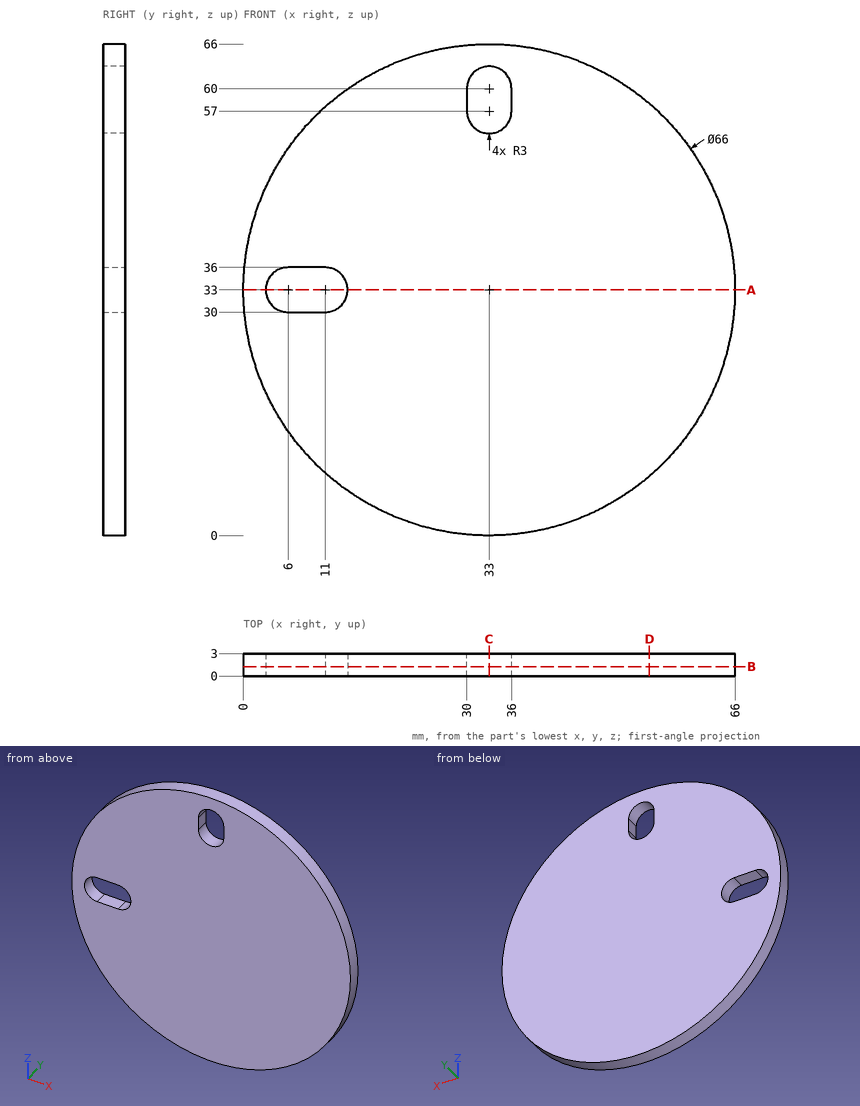
Geometry check sheet. Reference: drawing and pictorial views, mm from the part's lowest x, y, z. Coordinates: 2 decimals unless noted, no trailing zeros. Order: outer loops, then holes, each group sorted by start corner. A loop starts at its lowest first (then second) coordinate and runs counter-clockwise, first axis right, second up.
1. Sectioned sample at B-B, the plane y = 1.25. Record the cut outline in (x, z).
Results found:
outline: circle Ø66 at (33, 33); hole (6, 30) - (11, 30) arc R3 ccw to (11.04, 36) - (6, 36) arc R3 ccw to start; hole (30, 57) arc R3 ccw to (36, 57) - (36, 60) arc R3 ccw to (30, 60) - close
2. Sectioned sample at C-C, the plane x = 33. Record the cut outline in (y, z).
Results found:
outline: (0, 0) - (3, 0) - (3, 54) - (0, 54) - close; (0, 63) - (3, 63) - (3, 66) - (0, 66) - close
3. Sectioned sample at D-D, the plane x = 54.5. Record the cut outline in (y, z) (3 decimals).
Results found:
outline: (0, 7.965) - (3, 7.965) - (3, 58.035) - (0, 58.035) - close
4. Scan lines: line 1 (X direction, y = 2.1, z = 59.5) (1 decimal); line 2 (X direction, y = 1.5, z = 60) (1 decimal); line 3 (Z direction, x = 52, y = 2). Record each from-to range of solid material in increasing order.
Results found:
line 1: x = 13.3 to 30, 36 to 52.7
line 2: x = 14 to 30, 36 to 52
line 3: z = 6.02 to 59.98
5. Sectioned sample at A-A, the plane z = 33. Record the cut outline in (x, y).
Results found:
outline: (0, 0) - (3, 0) - (3, 3) - (0, 3) - close; (14, 0) - (66, 0) - (66, 3) - (14, 3) - close
6. Go/stop test with flat-tipped pins: pin 1 Ø1.5 at (y, z) = (1.5, 58.5) entering from -X; pin 2 Ø1.5 at (x, y) = (10, 2) entering from +Z; pin 3 Ø0.9 at (y, z) = (1.5, 58.5) entering from +X. Record where each tip stops, or that it passes through.
Results found:
pin 1: stops at x = 11.17
pin 2: stops at z = 57.37
pin 3: stops at x = 54.48
